Here's how the part is built. I have some questions about the finished solid (model axes, mm). Round coordinates to 2 decimals unless told otherwise and drop trailing zeros. Write each loop counter-clockwise with the first axis right and the second up, starting at its lowest first coordinate (ties: lowest second). Pieces come first, ordered by that corner, then holes. Notation, with made-up numbers: (45.25, 74.5) - (52.25, 74.5) arc R27 ccw to (52.25, 103.5) - close; hole circle Ø10 at (-22, -4). An arc over 180 degrees is marked (long way). Use one line per item in the form item = value. Start each with the question number.
1. We'd pull the mould along Y, two halves only. Please class faces 1 (the cylindrical face through (-38.169, 5.586, 0.402)), 2 (the cylindrical face through (38.169, -5.586, 0.402)), 3 (the flat face through (0, 7, 0)): +Y half, -Y half, draft (parallel to the pull), parting line (faces both ways), or undercut.
2. I want a section at B-B, the plane y = 2.25. List the corners of the cut face in (x, z) for me (3 decimals), plus the area to 3 significant figures.
3. I want a section at C-C, the plane z = 1.15. List the corners of the cut face in (x, y) for me, plus the area to 3 significant figures.
4. Will these pins go through, and if not, where does the flat tip stop? pin 1 (5 mm diameter, centred on x = 21, y = 6, fed in from -Z); pin 2 (2 mm diameter, centred on x = 39.69, y = 6.35, fed in from +Z).
5. I want a section at A-A, the plane x = -8. List the corners of the cut face in (y, z) for me, plus the area to 3 significant figures.
6. If I drill on line 1 along Y through (x, z) = (0, 0.35); line 2 along X through (y, z) = (3.5, 0.3) (3 decimals); line 3 along X through (y, z) = (3.25, 0.75), over which ranges is the centre line in solid material (lowest first)?
```python
from build123d import *

# Parameters (mm, degrees)
SKETCH1_W               = 82.55
SKETCH1_H               = 15.875
BOSS_EXTRUDE1_DEPTH     = 0.79375
SKETCH4_R               = 0.474599
BOSS_EXTRUDE2_DEPTH     = 0.635
MIRROR2_COPY_1_SKETCH_R = 0.474599
MIRROR2_COPY_1_DEPTH    = 0.635
CUT_EXTRUDE3_DEPTH      = 43.038786499
SKETCH7_R               = 0.6223
SKETCH7_R_2             = 0.6858
CUT_EXTRUDE4_DEPTH      = 43.05556869
FILLET1_R               = 1.1938
FILLET2_R               = 0.127


with BuildPart() as part:
    # Sketch1 → Boss-Extrude1 (new body)
    with BuildSketch(Plane.XY):
        Rectangle(SKETCH1_W, SKETCH1_H)
    extrude(amount=BOSS_EXTRUDE1_DEPTH)

    # Sketch4 → Boss-Extrude2 (add)
    with BuildSketch(Plane.XY.offset(0.79375)):
        with Locations((39.6875, 6.35)):
            Circle(SKETCH4_R)
    boss_extrude2 = extrude(amount=BOSS_EXTRUDE2_DEPTH)

    # Mirror1: Boss-Extrude2 across plane
    add(boss_extrude2.mirror(Plane.ZX))

    # Mirror2: Boss-Extrude2 across plane
    add(boss_extrude2.mirror(Plane(origin=(0, 0, 0), x_dir=(0, 0, 1), z_dir=(1, 0, 0))))

    # Mirror2 copy 1 sketch → Mirror2 copy 1 (add)
    with BuildSketch(Plane(origin=(0, 0, 0.79375), x_dir=(-1, 0, 0), z_dir=(0, 0, 1))):
        with Locations((39.6875, 6.35)):
            Circle(MIRROR2_COPY_1_SKETCH_R)
    extrude(amount=MIRROR2_COPY_1_DEPTH)

    # Sketch6 → Cut-Extrude3 (cut, through all)
    with BuildSketch(Plane.XY.offset(0.79375)):
        with BuildLine():
            Line((-36.35375, 6.35), (36.35375, 6.35))
            ThreePointArc((36.35375, 6.35), (38.149801224, 5.606051224), (38.89375, 3.81))
            Line((38.89375, 3.81), (38.89375, -3.81))
            ThreePointArc((38.89375, -3.81), (38.149801224, -5.606051224), (36.35375, -6.35))
            Line((36.35375, -6.35), (-36.35375, -6.35))
            ThreePointArc((-36.35375, -6.35), (-38.149801224, -5.606051224), (-38.89375, -3.81))
            Line((-38.89375, -3.81), (-38.89375, 3.81))
            ThreePointArc((-38.89375, 3.81), (-38.149801224, 5.606051224), (-36.35375, 6.35))
        make_face()
    extrude(amount=-CUT_EXTRUDE3_DEPTH, mode=Mode.SUBTRACT)

    # Sketch7 → Cut-Extrude4 (cut, through all)
    with BuildSketch(Plane.XY.offset(1.42875)):
        with Locations((-39.6875, 6.35)):
            Circle(SKETCH7_R)
        with Locations((39.6875, 6.35)):
            Circle(SKETCH7_R_2)
    extrude(amount=-CUT_EXTRUDE4_DEPTH, mode=Mode.SUBTRACT)

    # Fillet1
    fillet1_edges = [part.edges().sort_by_distance(p)[0] for p in [
        (41.275, -7.9375, 0.396875),
        (-41.275, -7.9375, 0.396875),
        (-41.275, 7.9375, 0.396875),
        (41.275, 7.9375, 0.396875),
    ]]
    fillet(fillet1_edges, radius=FILLET1_R)

    # Fillet2
    fillet2_edges = [part.edges().sort_by_distance(p)[0] for p in [
        (0, 7.9375, 0),
        (0, 7.9375, 0.79375),
        (41.275, 0, 0),
        (0, -7.9375, 0),
        (-41.275, 0, 0),
        (-40.925344075, 7.587844075, 0),
        (-40.925344075, -7.587844075, 0),
        (40.925344075, -7.587844075, 0),
        (40.925344075, 7.587844075, 0),
        (41.275, 0, 0.79375),
        (-41.275, 0, 0.79375),
        (0, -7.9375, 0.79375),
        (-40.925344075, 7.587844075, 0.79375),
        (-40.925344075, -7.587844075, 0.79375),
        (40.925344075, -7.587844075, 0.79375),
        (40.925344075, 7.587844075, 0.79375),
    ]]
    fillet(fillet2_edges, radius=FILLET2_R)


solid = part.part
```
Model answer:
q1.face_1 = undercut
q1.face_2 = undercut
q1.face_3 = draft
q2.outline = (-41.275, 0.127) arc R0.127 ccw to (-41.148, 0) - (-38.894, 0) - (-38.894, 0.794) - (-41.148, 0.794) arc R0.127 ccw to (-41.275, 0.667) - close; (38.894, 0) - (41.148, 0) arc R0.127 ccw to (41.275, 0.127) - (41.275, 0.667) arc R0.127 ccw to (41.148, 0.794) - (38.894, 0.794) - close
q2.area = 3.77 mm2
q3.outline = circle Ø0.95 at (-39.69, -6.35); circle Ø0.95 at (39.69, -6.35)
q3.area = 1.42 mm2
q4.pin_1 = 0
q4.pin_2 = 0.79
q5.outline = (-7.94, 0.13) arc R0.13 ccw to (-7.81, 0) - (-6.35, 0) - (-6.35, 0.79) - (-7.81, 0.79) arc R0.13 ccw to (-7.94, 0.67) - close; (6.35, 0) - (7.81, 0) arc R0.13 ccw to (7.94, 0.13) - (7.94, 0.67) arc R0.13 ccw to (7.81, 0.79) - (6.35, 0.79) - close
q5.area = 2.51 mm2
q6.line_1 = -7.94 to -6.35, 6.35 to 7.94
q6.line_2 = -41.275 to -38.894, 38.894 to 41.275
q6.line_3 = -41.24 to -38.89, 38.89 to 41.24
